```python
from build123d import *

# Parameters (mm, degrees)
BOSS_EXTRU_1_DEPTH  = 1
SKETCH1_R           = 6.5
BOSS_EXTRUDE1_DEPTH = 20


with BuildPart() as part:
    # Esquisse1 → Révolution1 (revolve)
    with BuildSketch(Plane.XY, mode=Mode.PRIVATE) as r_volution1_sk:
        with BuildLine():
            Line((0, 0), (5, 0))
            Line((5, 0), (14.396926208, 3.420201433))
            ThreePointArc((14.396926208, 3.420201433), (14.728803197, 3.934870166), (14.322587886, 4.393144497))
            Line((14.322587886, 4.393144497), (5, 1))
            Line((5, 1), (0, 1))
            Line((0, 1), (0, 0))
        make_face()
    revolve(r_volution1_sk.sketch.rotate(Axis((0, 0, 0), (0, 1, 0)), 90), axis=Axis((0, 0, 0), (0, 1, 0)))

    # Esquisse2 → Boss.-Extru.1 (add)
    with BuildSketch(Plane.XZ):
        Polygon((2.792425312, -4.14757289), (4.988116143, 0.344524813), (2.195690831, 4.492097703), (-2.792425312, 4.14757289), (-4.988116143, -0.344524813), (-2.195690831, -4.492097703), align=None)
    extrude(amount=BOSS_EXTRU_1_DEPTH)

    # Sketch1 → Boss-Extrude1 (add)
    with BuildSketch(Plane.XZ.offset(1)):
        with Locations(Location((0, 0, 0), (0, 0, 270))):
            Circle(SKETCH1_R)
    extrude(amount=BOSS_EXTRUDE1_DEPTH)


solid = part.part
```
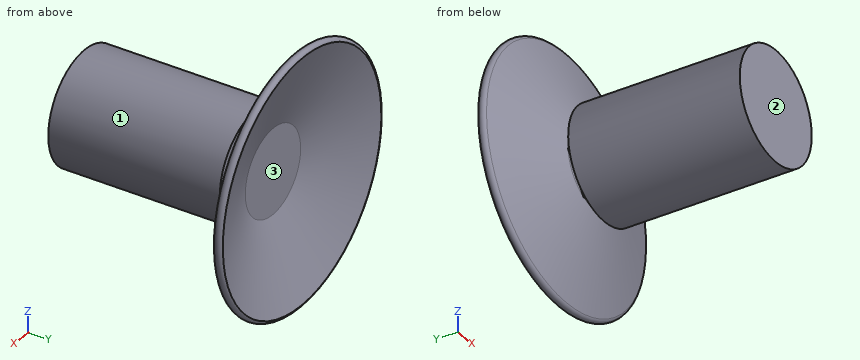
For this review, take the finished solid that the model builds, in its own axes (mm). Face numbers are marked on the shaded views. A direction names the side the tool comes from. Give positions to 0.01 mm unless a question says otherwise; leave off trailing zeros. Write each loop counter-clockwise with the first axis right and the second up, starting at its lowest first coordinate (ties: lowest second). Pieces come first, ordered by that corner, then holes.
Item 1: Take a section at B-B (y = -7.5). Give the boundary of the cut face in (x, z).
Item 2: Insertion check: P1, Ø1.5, axis at y = -18, z = 4.5, coming from the +X side; P2, Ø10, axis at x = -5.5, y = -15, coming from the -Z side; P3, Ø8, axis at x = 8.5, z = 5.5, coming from the +Y side. Each pin has a flat end and moves straight along its axis. Give the tip position at first contact, or say it passes through.
Item 3: Take a section at A-A (x = 0). Give the boundary of the cut face in (y, z).
Item 4: Machinability: for the marked faces 1, 2 and 3, which of the approach directions +Z, -Z, +X, -X, +Y, -Y give a long, thin tool a straight path to every point of the face, cutting with its end or side? Answer none if there is none.
Item 5: Wall thickness on probe 1 along X at (y, z) = (-17.75, -5); probe 2 along Y at (x, z) = (-2.5, 3); probe 3 along Y at (x, z) = (-4.25, -3): over which ranges is each line inside the solid? List them lowest first.
Established:
1. outline: circle Ø13 at (0, 0)
2. P1: stops at x = 5.31
2. P2: stops at z = -6.48
2. P3: stops at y = 4.32
3. outline: (-21, -6.5) - (-1, -6.5) - (-1, -4.34) - (0, -4.34) - (0, -5) - (3.42, -14.4) arc R0.51 ccw to (4.39, -14.32) - (1, -5) - (1, 5) - (4.39, 14.32) arc R0.51 ccw to (3.42, 14.4) - (0, 5) - (0, 4.34) - (-1, 4.34) - (-1, 6.5) - (-21, 6.5) - close
4. face 1: -Y
4. face 2: +Z, -Z, +X, -X, -Y
4. face 3: +Y
5. probe 1: x = -4.15 to 4.15
5. probe 2: y = -21 to 1
5. probe 3: y = -21 to -1, 0.07 to 1.07
